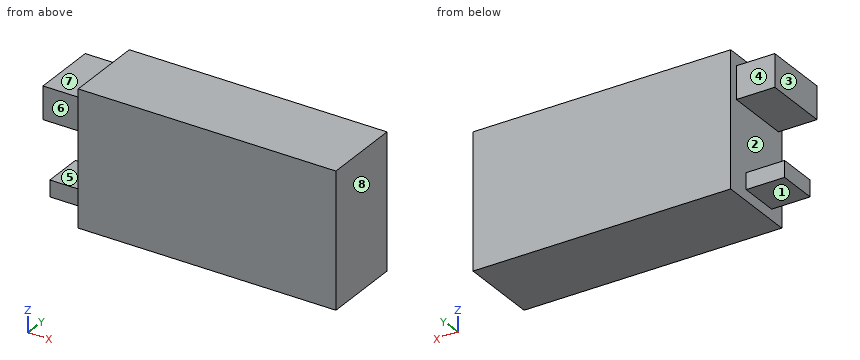
```python
from build123d import *

# Parameters (mm, degrees)
SKETCH1_W           = 67
SKETCH1_H           = 35
BOSS_EXTRUDE1_DEPTH = 20.6
SKETCH2_W           = 4.254648544
SKETCH2_H           = 10.285150392
SKETCH2_W_2         = 8.472300143
SKETCH2_H_2         = 17.018594174
BOSS_EXTRUDE2_DEPTH = 10


with BuildPart() as part:
    # Sketch1 → Boss-Extrude1 (new body)
    with BuildSketch(Plane(origin=(0, 0, 0), x_dir=(1, 0, 0), z_dir=(0, 1, 0))):
        Rectangle(SKETCH1_W, SKETCH1_H)
    extrude(amount=BOSS_EXTRUDE1_DEPTH)

    # Sketch2 → Boss-Extrude2 (add)
    with BuildSketch(Plane.ZY.offset(33.5)):
        with Locations((-12.560462439, 9.227088628)):
            Rectangle(SKETCH2_W, SKETCH2_H)
        with Locations((10.303648864, 9.81903973)):
            Rectangle(SKETCH2_W_2, SKETCH2_H_2)
    extrude(amount=BOSS_EXTRUDE2_DEPTH)


solid = part.part
```
Check sheet for the modelled part. Datum: model origin and axes. Units: mm. Face numbers are marked on the shaded views. A direction names the side the tool comes from. Round coordinates to 2 decimals unless told otherwise and drop trailing zeros. Order: outer loops, then holes, each group sorted by start corner. A loop starts at its lowest first (then second) coordinate and runs counter-clockwise, first axis right, second up.
1) Section check D-D (z = 2). Record the boundary of the cut face in (x, y).
2) Scan lines: line 1 (Z direction, x = -38, y = 16.5); line 2 (X direction, y = 14.5, z = -11). Record each from-to range of solid material in increasing order.
3) Section check A-A (z = 11.5). Record the boundary of the cut face in (x, y), and give its area (3 significant figures).
4) Go/stop test with flat-tipped pins: pin 1 Ø2 at (x, z) = (-36.5, -12) entering from +Y; pin 2 Ø3 at (x, y) = (-38, 6.5) entering from +Z; pin 3 Ø4 at (x, z) = (-37, 12) entering from +Y. Record where each tip stops, or that it passes through.
5) Tool access check on the marked faces 4, 5, 6, 7 and 8. Record the directions out of +Z, -Z, +X, -X, +Y, -Y that give a thin tool (end or side, any length) a straight path to the whole face; none if there is none.
6) Mould release check, pull along Z, two halves, no side actions. Record for the marked faces 1, 2 and 3: +Z half, -Z half, draft (parallel to the pull), parting line (faces both ways), or undercut.
7) Section check C-C (z = -12.5). Record the boundary of the cut face in (x, y).
8) Section check B-B (y = 8). Record the boundary of the cut face in (x, z).
Result:
1. outline: (-33.5, 0) - (33.5, 0) - (33.5, 20.6) - (-33.5, 20.6) - close
2. line 1: z = 6.07 to 14.54
2. line 2: x = -33.5 to 33.5
3. outline: (-43.5, 1.31) - (-33.5, 1.31) - (-33.5, 0) - (33.5, 0) - (33.5, 20.6) - (-33.5, 20.6) - (-33.5, 18.33) - (-43.5, 18.33) - close
3. area: 1,550 mm2
4. pin 1: stops at y = 14.37
4. pin 2: stops at z = 14.54
4. pin 3: stops at y = 18.33
5. face 4: +Z, -Z, -X, +Y
5. face 5: -X, +Y, -Y
5. face 6: +Z, -Z, -X, -Y
5. face 7: +Z, -X, +Y, -Y
5. face 8: +Z, -Z, +X, +Y, -Y
6. face 1: -Z half
6. face 2: undercut
6. face 3: draft
7. outline: (-43.5, 4.08) - (-33.5, 4.08) - (-33.5, 0) - (33.5, 0) - (33.5, 20.6) - (-33.5, 20.6) - (-33.5, 14.37) - (-43.5, 14.37) - close
8. outline: (-43.5, -14.69) - (-33.5, -14.69) - (-33.5, -17.5) - (33.5, -17.5) - (33.5, 17.5) - (-33.5, 17.5) - (-33.5, 14.54) - (-43.5, 14.54) - (-43.5, 6.07) - (-33.5, 6.07) - (-33.5, -10.43) - (-43.5, -10.43) - close
